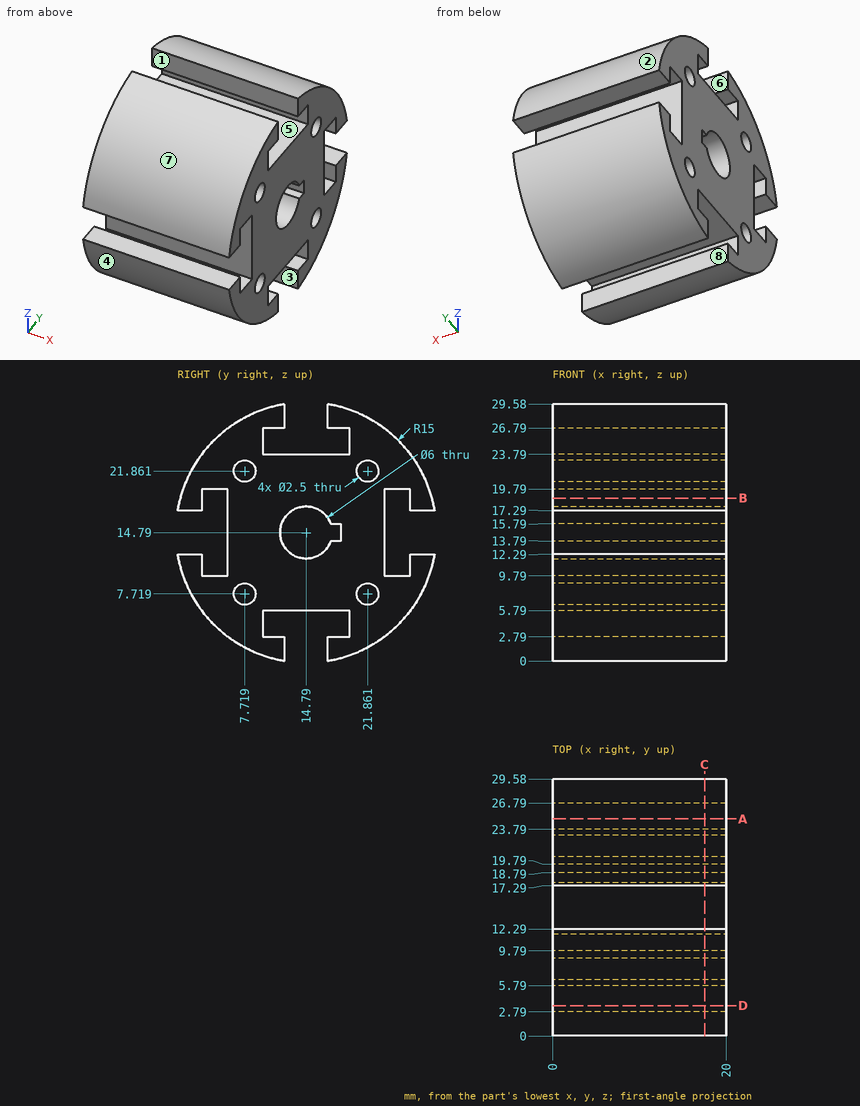
Study the drawing (mm; zero at the part's minimum x, y, z) and answer. A direction names the side the tool comes from. Coordinates: 2 decimals unless noted, no trailing zeros. Loops run counter-clockwise (first coordinate to the right, second up) from the corner with the lowest first, then second, coordinate; pieces in that order, holes last. Notation, with made-up numbers: M 63,24.5 L 117,24.5 A34 ccw 117,55.5 Z; hole C 57,-2 d6. An arc over 180 degrees is marked long. Answer in a Markdown table with one row per item. Add a question column.
1. A tool of negligible diameter and unlimited length cuts with its end or side. For the marked faces 5, 6, 7 and 8, from which of +Z, -Z, +X, -X, +Y, -Y can it reach the whole face along a straight path? Write none if from no direction.
2. Find section A-A, the plane y = 25. Write down the section's boundary in (x, z).
3. Find section B-B, the plane z = 18.75. Write down the section's boundary in (x, y), then the cut area to 3 significant figures.
4. Flat-ended cylindrical pins translate along their axes: P1, Ø3, axis at x = 11, y = 2, coming from the -Z side (1 decimal); P2, Ø8, axis at x = 12, y = 15, coming from the -Z side; P3, Ø3, axis at x = 17, y = 22.5, coming from the +Z side (1 decimal); P4, Ø10, axis at x = 9.5, y = 5, coming from the -Z side (1 decimal). Find the tip coordinate at first contact, or state that the pin passes through.
5. Find section D-D, the plane y = 3.5. Write down the section's boundary in (x, z) (1 decimal).
6. Find section C-C, the plane x = 17.5. State how many separate pieces and enclosed holes the cut face has, then the cut area to 3 significant figures.
7. The mould has two halves that part along Y. Classify the marked faces 1, 2, 3 and 4: pulls with the +Y half, pulls with the -Y half, needs draft (parallel to the pull), parting line crosses it, or undercut.
8. Consider L1, parallel to Z at x = 17, y = 21.75 (1 decimal); L2, parallel to Z at x = 5.75, y = 10.75 (1 decimal); L3, parallel to Y at x = 18.5, z = 8.5 (1 decimal). Determine where each line is inside the solid, lowest interval first.
Reported:
| question | item | result |
|---|---|---|
| 1 | face 5 | +X, -X |
| 1 | face 6 | +Z, +X, -X |
| 1 | face 7 | +Z, +X, -X, -Y |
| 1 | face 8 | -Z, +X, -X |
| 2 | outline | M 0,3.8 L 20,3.8 L 20,9.79 L 0,9.79 Z; M 0,19.79 L 20,19.79 L 20,25.78 L 0,25.78 Z |
| 3 | outline | M 0,0.32 L 20,0.32 L 20,2.79 L 0,2.79 Z; M 0,5.79 L 20,5.79 L 20,23.79 L 0,23.79 Z; M 0,26.79 L 20,26.79 L 20,29.26 L 0,29.26 Z |
| 3 | area | 459 mm^2 |
| 4 | P1 | stops at z = 4.9 |
| 4 | P2 | stops at z = 0 |
| 4 | P3 | stops at z = 28.4 |
| 4 | P4 | stops at z = 0.6 |
| 5 | outline | M 0,4.9 L 20,4.9 L 20,9.8 L 0,9.8 Z; M 0,19.8 L 20,19.8 L 20,24.7 L 0,24.7 Z |
| 6 | separate pieces | 1 |
| 6 | enclosed holes | 5 |
| 6 | area | 478 mm^2 |
| 7 | face 1 | undercut |
| 7 | face 2 | pulls with the +Y half |
| 7 | face 3 | undercut |
| 7 | face 4 | pulls with the -Y half |
| 8 | L1 | z = 1.5 to 6.5, 9 to 20.6, 23.1 to 28.1 |
| 8 | L2 | z = 0.3 to 2.8, 5.8 to 23.8, 26.8 to 29.2 |
| 8 | L3 | y = 1.2 to 6.7, 8.7 to 20.9, 22.8 to 28.4 |
